The model under review builds one solid part; all positions refer to its coordinate system, in mm. A direction names the side the tool comes from. Round coordinates to 2 decimals unless told otherwise and drop trailing zeros. Write each loop counter-clockwise with the first axis right and the second up, starting at its lowest first coordinate (ties: lowest second). Pieces come first, ordered by that corner, then holes. Notation, with made-up numbers: (31, 31) -> (86, 31) arc R11 ccw to (86, 35) -> close; hole circle Ø11 at (-35.75, 53). An arc over 180 degrees is marked (long way). Use CSV: the item, a comma, the result in double quotes. Start each with the question number.
1) Wall thickness on probe 1 along Z at (x, y) = (4, -31.5); probe 2 along X at (y, z) = (-13, 22.5); probe 3 along X at (y, z) = (2, 42): over which ranges is each line inside the solid? List them lowest first. Write a range as [from, to].
2) Take a section at A-A, the plane y = 0. Give the boundary of the cut face in (x, z).
3) Take a section at D-D, the plane z = 61.5. Give the boundary of the cut face in (x, y).
4) For pin 1 Ø6 at (y, z) = (-23, 50) entering from -X; pin 2 Ø12 at (y, z) = (-12, 42.5) entering from +X; pin 3 Ø3 at (y, z) = (-19, 58.5) entering from -X, all flat-tipped, find the tip position at first contact; note any pin that passes through.
5) Take a section at C-C, the plane z = 45. Give the boundary of the cut face in (x, y).
6) Mouldability with a two-part tool opening along Y and no side actions: class faces 3 (the face through (12, -19, 80)), 4 (the face through (-23.846, 7.509, 43.524)), 5 (the face through (0, 0, 10)) as released by +Y, released by -Y, zero draft, split by the parting line, or undercut.
7) Machinability: for faces 1 (the face through (-24, 8, 10)), 2 (the face through (1, 1, 0)), which of the approach directions +Z, -Z, +X, -X, +Y, -Y give a long, thin tool a straight path to every point of the face, cutting with its end or side? Answer none if there is none.
from build123d import *

# Parameters (mm, degrees)
F2_R = 2
F3_R = 5


with BuildPart() as f1:
    # F0 (on Front) → F1 (revolve)
    with BuildSketch(Plane.XZ):
        Polygon((-40, 0), (0, 0), (0, 10), (-15, 10), (-20, 80), (-25, 80), (-25, 10), (-40, 10), align=None)
    revolve(axis=Axis((0, 0, 5), (0, 0, -1)))

    # F2
    f2_edges = [f1.edges().sort_by_distance(p)[0] for p in [
        (15, 0, 10),
        (20, 0, 80),
        (25, 0, 80),
    ]]
    fillet(f2_edges, radius=F2_R)

    # F3
    f3_edges = [f1.edges().sort_by_distance(p)[0] for p in [
        (40, 0, 10),
    ]]
    fillet(f3_edges, radius=F3_R)


solid = f1.part
Values found:
1,probe 1,"[0, 10]"
1,probe 2,"[-21.35, -9.14], [9.14, 21.35]"
1,probe 3,"[-24.92, -17.17], [17.17, 24.92]"
2,outline,"(-40, 0) -> (40, 0) -> (40, 5) arc R5 ccw to (35, 10) -> (25, 10) -> (25, 78) arc R2 ccw to (23, 80) -> (21.86, 80) arc R2 ccw to (19.87, 78.14) -> (15.13, 11.86) arc R2 cw to (13.14, 10) -> (-13.14, 10) arc R2 cw to (-15.13, 11.86) -> (-19.87, 78.14) arc R2 ccw to (-21.86, 80) -> (-23, 80) arc R2 ccw to (-25, 78) -> (-25, 10) -> (-35, 10) arc R5 ccw to (-40, 5) -> close"
3,outline,"circle Ø50 at (0, 0); hole circle Ø37.36 at (0, 0)"
4,pin 1,"x = -15"
4,pin 2,"x = 24.27"
4,pin 3,"x = -17.85"
5,outline,"circle Ø50 at (0, 0); hole circle Ø35 at (0, 0)"
6,face 3,"zero draft"
6,face 4,"split by the parting line"
6,face 5,"undercut"
7,face 1,"+Z"
7,face 2,"-Z, +X, -X, +Y, -Y"
